Input: part model. Units: mm. Frame: model coordinates. Face numbers are marked on the shaded views. Coordinates: 2 decimals unless noted, no trailing zeros. Order: outer loops, then holes, each group sorted by start corner. A loop starts at its lowest first (then second) coordinate and runs counter-clockwise, first axis right, second up. Notation, with made-up numbers: (61, -32.5) -> (103, -32.5) arc R30 ccw to (103, 4.5) -> close; hole circle Ø1 at (-32.5, -19). An arc over 180 degrees is marked (long way). Use CSV: the item, a comma, the result in double quotes. Start each with the question number.
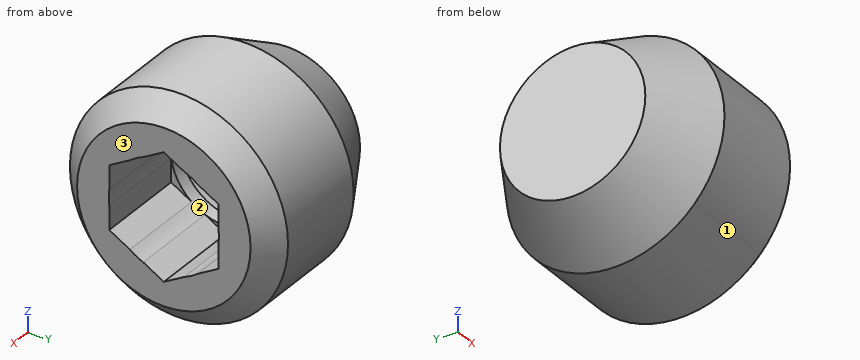
Autodesk Inventor part; units mm, degrees
ref_plane "Work Plane3" through (2.5, 0, 0) normal (0, -0.5, -0.866) x (1, 0, 0)
ref_plane "YZ Plane" through (0, 0, 0) normal (1, 0, 0) x (0, 1, 0)
ref_plane "XZ Plane" through (0, 0, 0) normal (0, 1, 0) x (-1, 0, 0)
sketch "Esquisse1" plane through (0, 0, 0) normal (0, 0, 1) x (1, 0, 0)
  line L0 (0, 0) -> (1.2503, 0)
  line L1 (5, 1.515) -> (5, 3)
  line L2 (5, 3) -> (0, 3)
  line L3 (5, 1.515) -> (2.125, 1.515)
  line L4 (2.125, 1.515) -> (1.2503, 0)
  line L5 (-1, 0) -> (6, 0)
  line L6 (0, 3) -> (0, 0)
  line L7 (0, -0.6) -> (0, 3.6)
  dimension "d0" = 2.875
  dimension "d1" = 60
  dimension "d2" = 6
  dimension "d3" = 3.03
  dimension "d12" = 5
revolve "Corps" add sketch "Esquisse1" angle 360 about axis through (0, 0, 0) along (1, 0, 0)
sketch "Esquisse2" plane through (5, 0, 0) normal (1, 0, 0) x (0, 0, -1)
  line L0 (-0.866, 1.5) -> (0.866, 1.5)
  line L1 (0.866, 1.5) -> (1.7321, 0)
  line L2 (1.7321, 0) -> (0.866, -1.5)
  line L3 (0.866, -1.5) -> (-0.866, -1.5)
  line L4 (-0.866, -1.5) -> (-1.7321, 0)
  line L5 (-1.7321, 0) -> (-0.866, 1.5)
  point P0 (0, 0)
  point P1 (0, 0)
  dimension "d13" = 3
extrude "Rainure" cut sketch "Esquisse2" against normal blind 2.5
thread "Filetage"
chamfer "Chanfrein1" distance 0.6135 angle 45 1 edges at (5, -3, 0) measured on face at (5, 1.628, -1.8837)
chamfer "Chanfrein2" distance 1 angle 60 1 edges at (0, -3, 0) measured on face at (0, -1.1424, 0.935)
ref_plane "Work Plane3" through (2.5, 0, 0) normal (0, -0.5, -0.866) x (1, 0, 0)
equation "\"d0\" = 1.15 * INTI"
equation "\"d2\" = NND"
equation "\"d3\" = 1.01 * SW"
equation "\"d12\" = NLG"
equation "\"d13\" = SW"
equation "\"d4\" = INTI"
equation "\"d8\" = -0.5 * GD1 + 0.5 * NND"
equation "\"d39\" = -0.5 * GD1 + 0.5 * NND"
equation "\"d15\" = -0.5 * SPD + 0.5 * NND"
equation "\"d40\" = -0.5 * SPD + 0.5 * NND"
equation "\"NND\" = 6"
equation "\"NLG\" = 5"
equation "\"INTI\" = 2.5"
equation "\"FAWI\" = 45deg"
equation "\"SW\" = 3"
equation "\"GD1\" = THREADDIA - 1.2269 * PTC"
equation "\"FAWI1\" = 30deg"
equation "\"SPD\" = 4"
equation "\"GUL\" = 0.61345 * PTC"
equation "\"TOA\" = 30deg"
equation "\"THREADDIA\" = 6"
equation "\"PTC\" = 1"
equation "\"GAL\" = 0.61345 * PTC"
equation "\"E0\" = 1.155 * SW"
properties part number "ANSI B18.3.6M - M6x1 x 5" material "Acier, doux"
1. Material intervals for line 1 along Y through (x, z) = (3.4, -1.15); line 2 along Y through (x, z) = (2.6, 0.55); line 3 along Z through (x, y) = (4.35, -0.25), sorted ascending.
2. Section A-A on x = 4.1. Return loops of the section in (y, z) (3 decimals), then the cut area to 3 significant figures.
3. Section B-B on x = 0.9. Return loops of the section in (y, z).
4. Contact query for a flat-ended pin moving along its axis: P1, Ø0.5, axis at x = 3, z = -0.5, coming from the -Y side. Output: stop coordinate, or through.
5. Pull-direction query (Y, two-part tool) for the marked faces 1, 2 and 3; classes: released by +Y, released by -Y, zero draft, split by the parting line, or undercut.
Values follow:
1,line 1,"y = -2.77 to -1.01, 1.01 to 2.77"
1,line 2,"y = -2.95 to -1.5, 1.5 to 2.95"
1,line 3,"z = -2.99 to -1.59, 1.59 to 2.99"
2,outline,"circle Ø6 at (0, 0); hole (-1.5, -0.866) -> (-0.934, -1.193) arc R1.515 ccw to (-0.566, -1.405) -> (0, -1.732) -> (0.566, -1.405) arc R1.515 ccw to (0.934, -1.193) -> (1.5, -0.866) -> (1.5, -0.213) arc R1.515 ccw to (1.5, 0.213) -> (1.5, 0.866) -> (0.934, 1.193) arc R1.515 ccw to (0.566, 1.405) -> (0, 1.732) -> (-0.566, 1.405) arc R1.515 ccw to (-0.934, 1.193) -> (-1.5, 0.866) -> (-1.5, 0.213) arc R1.515 ccw to (-1.5, -0.213) -> close"
2,area,"20.5 mm2"
3,outline,"circle Ø5.04 at (0, 0)"
4,P1,"stops at y = -2.99"
5,face 1,"split by the parting line"
5,face 2,"undercut"
5,face 3,"zero draft"
